from build123d import *

# Parameters (mm, degrees)
CYLINDER029_R       = 11.25
CYLINDER029_DEPTH   = 7
CYLINDER030_R       = 13
CYLINDER030_DEPTH   = 7
BOX009_W            = 58
BOX009_H            = 10
BOX009_DEPTH        = 3
CONE005_PITCH_ANGLE = 90
CYLINDER028_R       = 6
CYLINDER028_DEPTH   = 4
CYLINDER027_R       = 8
CYLINDER027_DEPTH   = 4
PAD003_DEPTH        = 15
SKETCH004_R         = 4.5
PAD004_DEPTH        = 20
CHAMFER004_SIZE     = 2
CHAMFER005_SIZE     = 2
FILLET003_R         = 5


with BuildPart() as obj1:
    # Cylinder029 → Cylinder029 (new body)
    with BuildSketch(Plane.XY):
        Circle(CYLINDER029_R)
    extrude(amount=CYLINDER029_DEPTH)


with BuildPart() as cut037:
    # Cylinder030 → Cylinder030 (new body)
    with BuildSketch(Plane.XY):
        Circle(CYLINDER030_R)
    extrude(amount=CYLINDER030_DEPTH)

    # Cut037: cut obj1
    add(obj1.part, mode=Mode.SUBTRACT)


with BuildPart() as cut037_1:
    # Cut037 placement: moved
    add(cut037.part.moved(Location((41, 30, 5))))


with BuildPart() as obj2:
    # Box009 → Box009 (new body)
    with BuildSketch(Plane(origin=(3, 0, 3), x_dir=(1, 0, 0), z_dir=(0, 0, 1))):
        with Locations((29, 5)):
            Rectangle(BOX009_W, BOX009_H)
    extrude(amount=BOX009_DEPTH)


with BuildPart() as cone_forat_cargol005:
    # Cone004 → Cone004 (revolve)
    with BuildSketch(Plane(origin=(55, 5, 0), x_dir=(1, 0, 0), z_dir=(0, -1, 0))):
        Polygon((0, 0), (3, 0), (1.75, 3), (0, 3), align=None)
    revolve(axis=Axis((55, 5, 0), (0, 0, 1)))


with BuildPart() as cone_forat_cargol004:
    # Cone003 → Cone003 (revolve)
    with BuildSketch(Plane(origin=(25, 5, 0), x_dir=(1, 0, 0), z_dir=(0, -1, 0))):
        Polygon((0, 0), (3, 0), (1.75, 3), (0, 3), align=None)
    revolve(axis=Axis((25, 5, 0), (0, 0, 1)))


with BuildPart() as cone_forat_cargol006:
    # Cone005 → Cone005 (revolve)
    with BuildSketch(Plane.XZ):
        Polygon((0, 0), (3, 0), (1.75, 3), (0, 3), align=None)
    revolve(axis=Axis((0, 0, 0), (0, 0, 1)))


with BuildPart() as cone_forat_cargol006_1:
    # Cone005 pitch: moved
    add(cone_forat_cargol006.part.rotate(Axis((0, 0, 0), (0, 1, 0)), CONE005_PITCH_ANGLE))


with BuildPart() as cone_forat_cargol006_2:
    # Cone005 placement: moved
    add(cone_forat_cargol006_1.part.moved(Location((0, 5, 10))))


with BuildPart() as cyl_brida_int005:
    # Cylinder028 → Cylinder028 (new body)
    with BuildSketch(Plane.XY):
        Circle(CYLINDER028_R)
    extrude(amount=CYLINDER028_DEPTH)


with BuildPart() as cyl_brida_ext005:
    # Cylinder027 → Cylinder027 (new body)
    with BuildSketch(Plane.XY):
        Circle(CYLINDER027_R)
    extrude(amount=CYLINDER027_DEPTH)


with BuildPart() as obj3:
    # Cut036 base: copy of Cyl-brida-ext005
    add(cyl_brida_ext005.part)

    # Cut036: cut Cyl-brida-int005
    add(cyl_brida_int005.part, mode=Mode.SUBTRACT)


with BuildPart() as obj3_1:
    # Cut036 placement: moved
    add(obj3.part.moved(Location((10, 30, 12))))


with BuildPart() as obj4:
    # Cut035 base: copy of Cyl-brida-ext005
    add(cyl_brida_ext005.part)

    # Cut035: cut Cyl-brida-int005
    add(cyl_brida_int005.part, mode=Mode.SUBTRACT)


with BuildPart() as obj4_1:
    # Cut035 placement: moved
    add(obj4.part.moved(Location((10, 30, 4))))


with BuildPart() as obj5:
    # Sketch003 → Pad003 (new body)
    with BuildSketch(Plane.XY.offset(5)):
        Polygon((3, 10), (21, 10), (21, 50), (61, 50), (61, 0), (3, 0), align=None)
    extrude(amount=PAD003_DEPTH)


with BuildPart() as y_end_idler:
    # Sketch004 → Pad004 (new body)
    with BuildSketch(Plane.XY):
        with BuildLine():
            ThreePointArc((6.75, 30), (11, 25.75), (15.25, 30))
            Line((15.25, 30), (21, 30))
            Line((21, 30), (21, 50))
            Line((21, 50), (61, 50))
            Line((61, 50), (61, 0))
            Line((0, 0), (61, 0))
            Line((0, 30), (0, 0))
            Line((6.75, 30), (0, 30))
        make_face()
        with Locations((41, 30)):
            Circle(SKETCH004_R, mode=Mode.SUBTRACT)
    extrude(amount=PAD004_DEPTH)

    # Cut034: cut obj5
    add(obj5.part, mode=Mode.SUBTRACT)

    # Cut033: cut obj4
    add(obj4_1.part, mode=Mode.SUBTRACT)

    # Cut032: cut obj3
    add(obj3_1.part, mode=Mode.SUBTRACT)

    # Cut030: cut Cone-forat-cargol006
    add(cone_forat_cargol006_2.part, mode=Mode.SUBTRACT)

    # Cut029: cut Cone-forat-cargol004
    add(cone_forat_cargol004.part, mode=Mode.SUBTRACT)

    # Cut028: cut Cone-forat-cargol005
    add(cone_forat_cargol005.part, mode=Mode.SUBTRACT)

    # Cut031: cut obj2
    add(obj2.part, mode=Mode.SUBTRACT)

    # Fusion002: union Cut037
    add(cut037_1.part)

    # Chamfer004
    chamfer004_edges = [y_end_idler.edges().sort_by_distance(p)[0] for p in [
        (21, 20, 5),
    ]]
    chamfer(chamfer004_edges, length=CHAMFER004_SIZE)

    # Chamfer005
    chamfer005_edges = [y_end_idler.edges().sort_by_distance(p)[0] for p in [
        (28, 30, 5),
    ]]
    chamfer(chamfer005_edges, length=CHAMFER005_SIZE)

    # Fillet003
    fillet003_edges = [y_end_idler.edges().sort_by_distance(p)[0] for p in [
        (61, 50, 2.5),
        (21, 50, 2.5),
    ]]
    fillet(fillet003_edges, radius=FILLET003_R)


with BuildPart() as part_mirroring001:
    # Part__Mirroring001: instance of y-end-idler
    add(y_end_idler.part.mirror(Plane(origin=(0, 0, 0), x_dir=(0, -1, 0), z_dir=(1, 0, 0))))


solid = part_mirroring001.part
Work out the finished part from the listing and answer in its coordinate system (mm). A direction names the side the tool comes from. Coordinates: 2 decimals unless noted, no trailing zeros. Loops run counter-clockwise (first coordinate to the right, second up) from the corner with the lowest first, then second, coordinate; pieces in that order, holes last. Notation, with made-up numbers: M 54.25,39.5 L 104.25,39.5 A17 cw 104.25,63.5 Z; hole C 61.5,11 d4. An arc over 180 degrees is marked long. Answer in a Markdown table with one row per item. Add a question column.
1. Flat-ended cylindrical pins translate along their axes: P1, Ø8, axis at y = 4, z = 13.5, coming from the -X side; P2, Ø8, axis at x = -42.5, y = 24, coming from the +Z side; P3, Ø3, axis at x = -28, y = 4, coming from the +Z side. Find the tip coordinate at first contact, or state that the pin passes through.
2. Find section C-C, the plane x = -41. Write down the section's boundary in (y, z), then the cut area to 4 significant figures.
3. Find section A-A, the plane z = 14.25. Write down the section's boundary in (x, y).
4. Find section B-B, the plane y = 5. Write down the section's boundary in (x, z), then the cut area to 3 significant figures.
5. Consider L1, parallel to Y at x = -41, z = 9.75; L2, parallel to Y at x = -41, z = 3.6; L3, parallel to Z at x = -58, y = 22. Determine where each line is inside the solid, lowest interval first.
6. The mould has two halves that part along Y. Classify faces 1 (the conical face through (-53.05, 5.09, 2.52)), 2 (the flat face through (-35, 40, 12)), 3 (the cylindrical face through (-28.013, 30.572, 9.465)): pulls with the +Y half, pulls with the -Y half, needs draft (parallel to the pull), parting line crosses it, or undercut.
7. A tool of negligible diameter and unlimited length cuts with its end or side. For faces 4 (the cylindrical face through (-10, 24, 14)), 5 (the flat face through (-21, 37, 2)), 6 (the cylindrical face through (-29.76, 30.49, 8.45)), 7 (the flat face through (-41, 50, 2)), 8 (the flat face through (-22, 20, 6)), from which of +Z, -Z, +X, -X, +Y, -Y can it reach the whole face along a straight path? Write none if from no direction.
8. Find section D-D, the plane z = 10. Write down the section's boundary in (x, y), then the cut area to 3 significant figures.
Reported:
| question | item | result |
|---|---|---|
| 1 | P1 | stops at x = -3 |
| 1 | P2 | stops at z = 5 |
| 1 | P3 | stops at z = 3 |
| 2 | outline | M 0,0 L 25.5,0 L 25.5,5 L 18.75,5 L 18.75,12 L 17,12 L 17,7 L 15,5 L 10,5 L 10,3 L 0,3 Z; M 34.5,0 L 50,0 L 50,5 L 45,5 L 43,7 L 43,12 L 41.25,12 L 41.25,5 L 34.5,5 Z |
| 2 | area | 213.5 mm^2 |
| 3 | outline | M -21,10 L -3,10 L -3,0 L 0,0 L 0,30 L -2,30 A8 cw -18,30 L -21,30 Z; M -16,30 A6 ccw -4,30 L -6.75,30 A4.25 cw -15.25,30 Z |
| 4 | outline | M -61,0 L -58,0 L -56.75,3 L -61,3 Z; M -53.25,3 L -52,0 L -28,0 L -26.75,3 Z; M -23.25,3 L -22,0 L 0,0 L 0,7 L -3,8.25 L -3,3 Z; M -3,11.75 L 0,13 L 0,20 L -3,20 Z |
| 4 | area | 191 mm^2 |
| 5 | L1 | y = 17 to 18.75, 41.25 to 43 |
| 5 | L2 | y = 10 to 25.5, 34.5 to 50 |
| 5 | L3 | z = 0 to 5 |
| 6 | face 1 | undercut |
| 6 | face 2 | needs draft |
| 6 | face 3 | parting line crosses it |
| 7 | face 4 | none |
| 7 | face 5 | +Z, -Z, +X, +Y |
| 7 | face 6 | +Z |
| 7 | face 7 | +Z, -Z, +X, -X, +Y |
| 7 | face 8 | +Z, +Y, -Y |
| 8 | outline | C -41,30 d26; M -21,10 L -3,10 L -3,6.75 L 0,8 L 0,30 L -6.75,30 A4.25 cw -15.25,30 L -21,30 Z; M -3,0 L 0,0 L 0,2 L -3,3.25 Z; hole C -41,30 d22.5 |
| 8 | area | 541 mm^2 |
